Autodesk Inventor part; units mm, degrees
ref_plane "YZ Plane" through (0, 0, 0) normal (1, 0, 0) x (0, 1, 0)
ref_plane "XZ Plane" through (0, 0, 0) normal (0, 1, 0) x (-1, 0, 0)
ref_plane "XY Plane" through (0, 0, 0) normal (0, 0, 1) x (1, 0, 0)
sketch "Эскиз1" plane through (0, 0, 0) normal (0, 1, 0) x (-1, 0, 0)
  line L0 (-25, 25) -> (25, 25)
  line L1 (25, 25) -> (25, -25)
  line L2 (25, -25) -> (-25, -25)
  line L3 (-25, -25) -> (-25, 25)
  line L4 (-25, 25) -> (25, -25) construction
  line L5 (25, 25) -> (-25, -25) construction
  line L6 (-11.5, -5) -> (11.5, -5)
  line L7 (11.5, -5) -> (11.5, 5)
  line L8 (11.5, 5) -> (-11.5, 5)
  line L9 (-11.5, 5) -> (-11.5, -5)
  line L10 (-11.5, -5) -> (11.5, 5) construction
  line L11 (11.5, -5) -> (-11.5, 5) construction
  line L12 (-3.5, 5) -> (-3.5, -5)
  line L13 (4, 5) -> (4, -5) construction
  circle A0 centre (4, 0) radius 5
  point P0 (0, 0)
  point P1 (4, -5)
  point P2 (4, 5)
  dimension "d0" = 50
  dimension "d1" = 50
  dimension "d2" = 23
  dimension "d3" = 10
  dimension "d4" = 8
  dimension "d29" = 7.5
  dimension "d30" = 10
extrude "Выдавливание13" add sketch "Эскиз1" along normal blind 15
sketch "Эскиз6" plane through (0, 0, 0) normal (0, -1, 0) x (1, 0, 0)
  line L0 (22.5, 22.5) -> (-22.5, 22.5)
  line L1 (-22.5, 22.5) -> (-22.5, -22.5)
  line L2 (-22.5, -22.5) -> (22.5, -22.5)
  line L3 (22.5, -22.5) -> (22.5, 22.5)
  line L4 (22.5, 22.5) -> (-22.5, -22.5) construction
  line L5 (-22.5, 22.5) -> (22.5, -22.5) construction
  point P0 (0, 0)
  dimension "d41" = 45
  dimension "d42" = 45
extrude "Выдавливание14" add sketch "Эскиз6" along normal blind 5
extrude "Выдавливание15" cut sketch "Эскиз1" against normal through all contours L12 L8 A0 L6 | A0 L8 L7 L6 | A0
sketch "Эскиз7" plane through (0, 15, 0) normal (0, 1, 0) x (1, 0, 0)
  circle A0 centre (-4.0005, 0) radius 6.5
  line L0 (25, 25) -> (-25, 25)
  line L1 (-25, 25) -> (-25, -25)
  point P0 (0, 0)
  dimension "d47" = 13
  dimension "d48" = 25
  dimension "d49" = 20.9995
extrude "Выдавливание16" cut sketch "Эскиз7" against normal blind 15
properties part number "platform"
For this review, take the finished solid that the model builds, in its own axes (mm). A direction names the side the tool comes from. Coordinates: 2 decimals unless noted, no trailing zeros. Write each loop counter-clockwise with the first axis right and the second up, starting at its lowest first coordinate (ties: lowest second). Pieces come first, ordered by that corner, then holes. Notation, with made-up numbers: (1, -6) -> (35, -6) arc R10 cw to (35, -2) -> close; hole circle Ø1 at (84, 48). An arc over 180 degrees is marked (long way). Write each question's results on one line, items separated by ' | '. Start each with the question number.
1) Consider section B-B (y = -1.25). Write out the cut boundary in (x, z).
2) Consider section C-C (z = 3). Write out the cut boundary in (x, y).
3) Consider section A-A (x = -9). Write out the cut boundary in (y, z).
4) Wall thickness on L1, parallel to X at y = 11.75, z = -3; L2, parallel to Z at x = 9.5, y = 12; L3, parallel to Z at x = 20.5, y = -1: over which ranges is each line inside the solid? List them lowest first. Write a range as [from, to].
5) Insertion check: pin 1 (1.5 mm diameter, centred on x = -10, y = -3, fed in from -Z); pin 2 (2.5 mm diameter, centred on y = -3.5, z = 2.5, fed in from -X); pin 3 (2.5 mm diameter, centred on x = 8, z = 1, fed in from +Y). Each pin has a flat end and moves straight along its axis. Give the tip position at first contact, or say it passes through.
6) Consider section D-D (z = 19.5). Write out the cut boundary in (x, y).
7) For faces 5 (the face through (-25, 7, 0)), 6 (the face through (-11.5, 5, 0)), 7 (the face through (-3.9, 7.6, -6.5)), list the 3-axis set-ups (+Z, -Z, +X, -X, +Y, -Y) from which the entire face can be reached by the end or side of a thin tool; tool diameter is ignored.
8) The part is to be moulded in two halves that separate along Z. For faces 1 (the face through (0, -2, 22.5)), 2 (the face through (0, -2, -22.5)), 3 (the face through (-22.5, -2, 0)), 4 (the face through (-4, 0, 6)), say which applies: +Z half, -Z half, draft (parallel to the pull), parting line (faces both ways), or undercut.
Geometry says:
1) outline: (-22.5, -22.5) -> (22.5, -22.5) -> (22.5, 22.5) -> (-22.5, 22.5) -> close; hole (-11.5, -5) -> (3.5, -5) -> (3.5, 5) -> (-11.5, 5) -> close
2) outline: (-25, 0) -> (-22.5, 0) -> (-22.5, -5) -> (-11.5, -5) -> (-11.5, 15) -> (-25, 15) -> close; (3.5, -5) -> (22.5, -5) -> (22.5, 0) -> (25, 0) -> (25, 15) -> (11.5, 15) -> (11.5, 0) -> (3.5, 0) -> close
3) outline: (-5, -22.5) -> (0, -22.5) -> (0, -25) -> (15, -25) -> (15, -5) -> (-5, -5) -> close; (-5, 5) -> (15, 5) -> (15, 25) -> (0, 25) -> (0, 22.5) -> (-5, 22.5) -> close
4) L1: [-25, -11.5], [11.5, 25] | L2: [-25, -5], [5, 25] | L3: [-22.5, 22.5]
5) pin 1: z = -22.5 | pin 2: x = -22.5 | pin 3: y = 0
6) outline: (-25, 0) -> (-22.5, 0) -> (-22.5, -5) -> (22.5, -5) -> (22.5, 0) -> (25, 0) -> (25, 15) -> (-25, 15) -> close
7) face 5: +Z, -Z, -X, +Y, -Y | face 6: +Y, -Y | face 7: +Y
8) face 1: +Z half | face 2: -Z half | face 3: draft | face 4: undercut
